Autodesk Inventor part; units mm, degrees
ref_plane "YZ Plane" through (0, 0, 0) normal (1, 0, 0) x (0, 1, 0)
ref_plane "XZ Plane" through (0, 0, 0) normal (0, 1, 0) x (-1, 0, 0)
ref_plane "XY Plane" through (0, 0, 0) normal (0, 0, 1) x (1, 0, 0)
sketch "Sketch1" plane through (0, 0, 0) normal (0, 1, 0) x (-1, 0, 0)
  circle A0 centre (0, 0) radius 11
  dimension "d0" = 22
extrude "Extrusion1" add sketch "Sketch1" along normal blind 550
sketch "Sketch7" plane through (0, 550, 0) normal (0, 1, 0) x (1, 0, 0)
  circle A0 centre (0, 0) radius 10.2
  dimension "d23" = 20.4
extrude "Extrusion3" cut sketch "Sketch7" against normal through all
sketch "Sketch8" plane through (0, 0, 0) normal (0, -1, 0) x (1, 0, 0)
  circle A0 centre (0, 0) radius 11
  point P0 (0, 11)
ref_plane "Work Plane3" through (0, 0, 11) normal (0, 0, 1) x (1, 0, 0)
sketch "Sketch9" plane through (0, 0, 11) normal (0, 0, 1) x (1, 0, 0)
  arc A0 (10, 5) -> (-10, 5) centre (0, 5) ccw
  line L0 (-10, 5) -> (-10, 0)
  line L1 (11, 0) -> (-11, 0)
  line L2 (10, 5) -> (10, 0)
  point P0 (0, 0)
  dimension "d26" = 5
  dimension "d27" = 20
extrude "Extrusion4" cut sketch "Sketch9" against normal through all
sketch "Sketch10" plane through (0, 0, 0) normal (0, -1, 0) x (1, 0, 0)
  circle A0 centre (0, 0) radius 11
  point P0 (11, 0)
ref_plane "Work Plane4" through (11, 0, 0) normal (1, 0, 0) x (0, 1, 0)
sketch "Sketch11" plane through (11, 0, 0) normal (1, 0, 0) x (0, 1, 0)
  line L0 (0, -4.5826) -> (0, 4.5826)
  point P0 (0, 0)
  point P1 (5, 0)
  point P2 (0, 0)
  dimension "d30" = 5
hole "Hole3" at (11, 5, 0) direction (-1, 0, 0) diameter 3.4587 end through all
equation "\"d36\" = Thickness"
equation "\"BendRadius\" = Thickness"
equation "\"BendReliefWidth\" = Thickness"
equation "\"BendReliefDepth\" = 0.5 * Thickness"
equation "\"CornerReliefSize\" = 4 * Thickness"
equation "\"MinimumRemnant\" = 2 * Thickness"
equation "\"TransitionRadius\" = BendRadius"
equation "\"JacobiRadiusSize\" = BendRadius"
equation "\"GapSize\" = Thickness"
properties part number "Output link body"
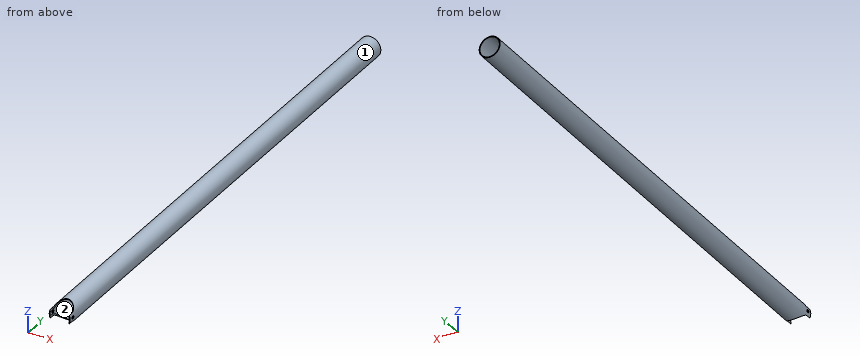
Build history of the part. All positions in model axes, mm. Face numbers are marked on the shaded views. Coordinates: 2 decimals unless noted, no trailing zeros. Order: outer loops, then holes, each group sorted by start corner. A loop starts at its lowest first (then second) coordinate and runs counter-clockwise, first axis right, second up. Notation, with made-up numbers: (63, 25) -> (101, 25) arc R9 cw to (101, 29) -> close; hole circle Ø10 at (17, 5.5). An arc over 180 degrees is marked (long way). Answer in a Markdown table with one row per item. Add a question column.
Q1. Drop flat-ended pins along their axis: pin 1 (1.3 mm diameter, centred on y = 2, z = 3.5, fed in from +X); pin 2 (12 mm diameter, centred on y = 147.5, z = -7, fed in from -X); pin 3 (1.5 mm diameter, centred on x = -4.5, y = 114, fed in from -Z); pin 4 (3 mm diameter, centred on x = 0.5, y = 273, fed in from +Z). Give the stop position or say it passes through.
Q2. Mould opens along X. For the marked faces 1 and 2 say: +X half, -X half, draft (parallel to the pull), parting line (faces both ways), or undercut.
Q3. Wall check: line 1 along X through (y, z) = (55.5, -0.5); line 2 along Z through (x, y) = (1, 425); line 3 along Y through (x, z) = (10.3, 0). Give the ranges that are in metal, low to high. Write a range as [from, to].
Q4. Band-saw the part on A-A, the plane x = 0. List the corners of the cut face in (y, z), then the cut area to 3 significant figures.
Answers follow:
| question | item | result |
|---|---|---|
| 1 | pin 1 | x = 10.62 |
| 1 | pin 2 | x = -10.95 |
| 1 | pin 3 | z = -10.34 |
| 1 | pin 4 | z = 11 |
| 2 | face 1 | parting line |
| 2 | face 2 | undercut |
| 3 | line 1 | [-10.99, -10.19], [10.19, 10.99] |
| 3 | line 2 | [-10.95, -10.15], [10.15, 10.95] |
| 3 | line 3 | [0, 3.27], [6.73, 550] |
| 4 | outline | (15, -11) -> (550, -11) -> (550, -10.2) -> (15, -10.2) -> close; (15, 10.2) -> (550, 10.2) -> (550, 11) -> (15, 11) -> close |
| 4 | area | 856 mm^2 |
